```python
from build123d import *

# Parameters (mm, degrees)
SKETCH_W     = 2
SKETCH_H     = 58
PAD_DEPTH    = 1
SKETCH001_W  = 2
SKETCH001_H  = 1.5
PAD001_DEPTH = 3
SKETCH002_W  = 2
SKETCH002_H  = 1.3
PAD002_DEPTH = 1
SKETCH003_W  = 2
SKETCH003_H  = 1.3
PAD003_DEPTH = 1


with BuildPart() as part:
    # Sketch → Pad (new body)
    with BuildSketch(Plane.XY):
        with Locations((1, 29)):
            Rectangle(SKETCH_W, SKETCH_H)
    extrude(amount=PAD_DEPTH)

    # Sketch001 (on Face6 of Pad) → Pad001 (join)
    with BuildSketch(Plane.XY.offset(1)):
        with Locations((1, 0.75)):
            Rectangle(SKETCH001_W, SKETCH001_H)
        with Locations((1, 57.25)):
            Rectangle(SKETCH001_W, SKETCH001_H)
    extrude(amount=PAD001_DEPTH)

    # Sketch002 (on Face14 of Pad001) → Pad002 (join)
    with BuildSketch(Plane.XZ.offset(-56.5)):
        with Locations((1, 3.35)):
            Rectangle(SKETCH002_W, SKETCH002_H)
    extrude(amount=PAD002_DEPTH)

    # Sketch003 (on Face17 of Pad002) → Pad003 (join)
    with BuildSketch(Plane(origin=(0, 1.5, 0), x_dir=(-1, 0, 0), z_dir=(0, 1, 0))):
        with Locations((-1, 3.35)):
            Rectangle(SKETCH003_W, SKETCH003_H)
    extrude(amount=PAD003_DEPTH)


solid = part.part
```
Could you check a few things on this model? Use its own coordinates, in mm. A direction names the side the tool comes from. Round coordinates to 2 decimals unless told otherwise and drop trailing zeros. Loops run counter-clockwise (first coordinate to the right, second up) from the corner with the lowest first, then second, coordinate; pieces in that order, holes last. Notation, with made-up numbers: (-39.5, 13.25) - (11.5, 13.25) arc R27 ccw to (11.5, 31.25) - close; hole circle Ø1 at (16, 3.5). An arc over 180 degrees is marked (long way). Answer as CSV lines item,"result".
1. On a 3-axis mill with a long thin cutter (end or side, diameter ignored), from which of +Z, -Z, +X, -X, +Y, -Y can I reach the whole of each face in a straight line? I mean faces 4 (the face through (1, 58, 2)), 5 (the face through (1, 55.5, 3)), 6 (the face through (1, 56, 2.7)). Say none if no direction works.
Filled in:
face 4,"+Z, -Z, +X, -X, +Y"
face 5,"+Z, +X, -X"
face 6,"+X, -X"
2. We'd pull the mould along Z, two halves only. Please class faces 1 (the face through (1, 1, 4)), 2 (the face through (2, 28.9, 0.8)), 3 (the face through (1, 2, 2.7)): +Z half, -Z half, draft (parallel to the pull), parting line (faces both ways), or undercut.
Filled in:
face 1,"+Z half"
face 2,"draft"
face 3,"undercut"
3. Please list where these lines run through material, in increasing order: line 1 along Y through (x, z) = (0.7, 2.1); line 2 along Y through (x, z) = (1.4, 3.4); line 3 along Z through (x, y) = (1.7, 43.5). Write a range as [from, to].
Filled in:
line 1,"y = [0, 1.5], [56.5, 58]"
line 2,"y = [0, 2.5], [55.5, 58]"
line 3,"z = [0, 1]"
4. I want a section at B-B on x = 1.4. List the corners of the cut face in (y, z) for me, then the cut area to 3 significant figures.
Filled in:
outline,"(0, 0) - (58, 0) - (58, 4) - (55.5, 4) - (55.5, 2.7) - (56.5, 2.7) - (56.5, 1) - (1.5, 1) - (1.5, 2.7) - (2.5, 2.7) - (2.5, 4) - (0, 4) - close"
area,"69.6 mm^2"
5. I want a section at A-A on z = 3.5. List the corners of the cut face in (x, y) for me, then the cut area to 3 significant figures.
Filled in:
outline,"(0, 0) - (2, 0) - (2, 2.5) - (0, 2.5) - close; (0, 55.5) - (2, 55.5) - (2, 58) - (0, 58) - close"
area,"10.0 mm^2"
6. I want a section at C-C on y = 33. List the corners of the cut face in (x, z) for me.
Filled in:
outline,"(0, 0) - (2, 0) - (2, 1) - (0, 1) - close"
7. For pin 1 Ø0.5 at (x, z) = (1.5, 1.5) entering from -Y, with a flat end and sliding along its axis, tell me the tip position at first contact or that it passes through.
Filled in:
pin 1,"stops at y = 0"
